Input: part model. Units: mm. Frame: model coordinates. Face numbers are marked on the shaded views. A direction names the side the tool comes from. Round coordinates to 2 decimals unless told otherwise and drop trailing zeros. Use one line per item in the form item = value. Start each with the question number.
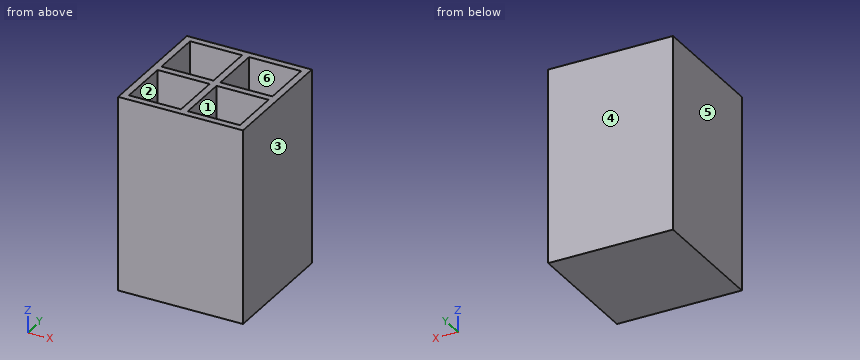
```python
from build123d import *

# Parameters (mm, degrees)
F0_W     = 57.15
F0_H     = 88.9
F1_DEPTH = 57.15
F2_W     = 23.8125
F2_H     = 23.8125
F6_DEPTH = 44.451
F3_W     = 23.8125
F3_H     = 23.8125
F7_DEPTH = 44.451
F4_W     = 23.8125
F4_H     = 23.8125
F8_DEPTH = 44.451
F5_W     = 23.8125
F5_H     = 23.8125
F9_DEPTH = 44.451


with BuildPart() as f1:
    # F0 (on Front) → F1 (new body)
    with BuildSketch(Plane.XZ):
        Rectangle(F0_W, F0_H)
    extrude(amount=F1_DEPTH)

    # F2 (on Top) → F6 (cut, through all)
    with BuildSketch(Plane.XY):
        with Locations((-13.49375, -15.08125)):
            Rectangle(F2_W, F2_H)
    extrude(amount=F6_DEPTH, mode=Mode.SUBTRACT)

    # F3 (on Top) → F7 (cut, through all)
    with BuildSketch(Plane.XY):
        with Locations((-13.49375, -42.06875)):
            Rectangle(F3_W, F3_H)
    extrude(amount=F7_DEPTH, mode=Mode.SUBTRACT)

    # F4 (on Top) → F8 (cut, through all)
    with BuildSketch(Plane.XY):
        with Locations((13.49375, -15.08125)):
            Rectangle(F4_W, F4_H)
    extrude(amount=F8_DEPTH, mode=Mode.SUBTRACT)

    # F5 (on Top) → F9 (cut, through all)
    with BuildSketch(Plane.XY):
        with Locations((13.49375, -42.06875)):
            Rectangle(F5_W, F5_H)
    extrude(amount=F9_DEPTH, mode=Mode.SUBTRACT)


solid = f1.part
```
Item 1: Draft query along X for the marked faces 1, 2, 3 and 4. Return one class per face: +X half, -X half, draft (parallel to the pull), parting line (faces both ways), or undercut.
Item 2: Reachability of the marked faces 5 and 6 from +Z, -Z, +X, -X, +Y, -Y: full face, straight path, thin tool, end or side. Return the list, or none.
Item 3: First-contact query: pin 1 (19 mm diameter, centred on x = -11.5, y = -45.5, fed in from +Z); pin 2 (1.5 mm diameter, centred on x = 22, y = -50, fed in from +Z). Flat tips, straight axial feed; report the tip coordinate or a pass-through.
Item 4: Ray query, line 1 (X direction, y = -9, z = 13.5) (1 decimal); line 2 (Z direction, x = -20, y = -10). Return the intervals inside material, ascending. Write a range as from..to.
Item 5: Cut plane B-B (z = 24.5). Give the number of separate pieces and of enclosed holes in the cut face, plus the area to 3 significant figures.
Final values:
q1.face_1 = undercut
q1.face_2 = undercut
q1.face_3 = +X half
q1.face_4 = draft
q2.face_5 = +Z, -Z, -X, +Y, -Y
q2.face_6 = +Z
q3.pin_1 = 44.45
q3.pin_2 = 0
q4.line_1 = -28.6..-25.4, -1.6..1.6, 25.4..28.6
q4.line_2 = -44.45..0
q5.separate_pieces = 1
q5.enclosed_holes = 4
q5.area = 998 mm^2
